Here's how the part is built. I have some questions about the finished solid (model axes, mm). A direction names the side the tool comes from. Round coordinates to 2 decimals unless told otherwise and drop trailing zeros. Order: outer loops, then holes, each group sorted by start corner. A loop starts at its lowest first (then second) coordinate and runs counter-clockwise, first axis right, second up. Notation, with made-up numbers: M -25.5,85.5 L -2.5,85.5 A34 ccw -2.5,121.5 Z; hole C -8.5,68 d7. An arc over 180 degrees is marked long. Write item = value, one per line. Start each with the question number.
Item 1: Please list where these lines run through material, in increasing order: L1, parallel to Z at x = 20.5, y = 8.5; L2, parallel to Z at x = 49, y = 0.5; L3, parallel to Y at x = -49, z = -0.75.
Item 2: I'm going to push flat-ended pins straight in: P1, Ø5, axis at x = 41.5, y = 10.5, coming from the +Z side; P2, Ø1.5, axis at x = 2, z = 2, coming from the +Y side; P3, Ø12, axis at x = 26, z = 6.5, coming from the +Y side. Where does each tip first touch, or does it pass through?
Item 3: We'd pull the mould along X, two halves only. Please class faces 1 (the face through (-35.76, 0, -11)), 2 (the face through (74.736, 9.446, -0.416)), 3 (the face through (40.76, 0, -11)), 4 (the face through (-100, 0, 0)): pulls with the +X half, pulls with the -X half, needs draft (parallel to the pull), parting line crosses it, or undercut.
Item 4: I want a section at A-A, the plane x = 11.5. List the corners of the cut face in (y, z) for me, plus the area to 3 significant figures.
Item 5: For faces 5 (the face through (100, 0, 0)), 6 (the face through (-40.76, 0, -11)), which set-ups out of +Z, -Z, +X, -X, +Y, -Y let a thin tool reach every point of the face, with its end or its side?
```python
from build123d import *
from OCP.BRepFilletAPI import BRepFilletAPI_MakeChamfer

# Parameters (mm, degrees)
CHAMFER_1_SIZE  = 0.5
CHAMFER_1_SIZE2 = 0.616401526


with BuildPart() as part:
    # 草图1 → 旋转1 (revolve)
    with BuildSketch(Plane.XY, mode=Mode.PRIVATE) as revolve_1_sk:
        Polygon((-100, 0), (100, 0), (100, 5), (50.759612349, 13.682408883), (40.759612349, 13.682408883), (40.759612349, 10.682408883), (35.759612349, 10.682408883), (35.759612349, 13.682408883), (-35.759612349, 13.682408883), (-35.759612349, 10.682408883), (-40.759612349, 10.682408883), (-40.759612349, 13.682408883), (-50.759612349, 13.682408883), (-100, 5), align=None)
    revolve(revolve_1_sk.sketch.rotate(Axis((-100, 0, 0), (1, 0, 0)), 180), axis=Axis((-100, 0, 0), (1, 0, 0)))

    # 倒角1: one chamfer whose edges measure the first distance from different faces: ONE call of the kernel's chamfer builder (chamfer() names one face for all edges)
    chamfer_1_edges_1 = [part.edges().sort_by_distance(p)[0] for p in [
        (100, 5, 0),
    ]]
    chamfer_1_side_1 = [part.faces().sort_by_distance(p)[0] for p in [
        (100, 0, 0),
    ]]
    chamfer_1_edges_2 = [part.edges().sort_by_distance(p)[0] for p in [
        (40.759612349, 13.682408883, 0),
        (35.759612349, 13.682408883, 0),
        (-35.759612349, 13.682408883, 0),
        (-40.759612349, 13.682408883, 0),
    ]]
    chamfer_1_edges_3 = [part.edges().sort_by_distance(p)[0] for p in [
        (-100, 5, 0),
    ]]
    chamfer_1_side_3 = [part.faces().sort_by_distance(p)[0] for p in [
        (-75.379806175, 9.341204442, 0),
    ]]
    chamfer_1 = BRepFilletAPI_MakeChamfer(part.part.solid().wrapped)
    for e in chamfer_1_edges_1:
        chamfer_1.Add(CHAMFER_1_SIZE, CHAMFER_1_SIZE2, e.wrapped, chamfer_1_side_1[0].wrapped)  # the first distance lies on this face
    for e in chamfer_1_edges_2:
        chamfer_1.Add(CHAMFER_1_SIZE, e.wrapped)
    for e in chamfer_1_edges_3:
        chamfer_1.Add(CHAMFER_1_SIZE, CHAMFER_1_SIZE2, e.wrapped, chamfer_1_side_3[0].wrapped)  # the first distance lies on this face
    add(Compound.cast(chamfer_1.Shape()), mode=Mode.REPLACE)


solid = part.part
```
Filled in:
q1.L1 = -10.72 to 10.72
q1.L2 = -13.67 to 13.67
q1.L3 = -13.66 to 13.66
q2.P1 = 11.1
q2.P2 = 13.63
q2.P3 = 13.67
q3.face_1 = undercut
q3.face_2 = pulls with the +X half
q3.face_3 = undercut
q3.face_4 = pulls with the -X half
q4.outline = C 0,0 d27.36
q4.area = 588 mm^2
q5.face_5 = +Z, -Z, +X, +Y, -Y
q5.face_6 = none
